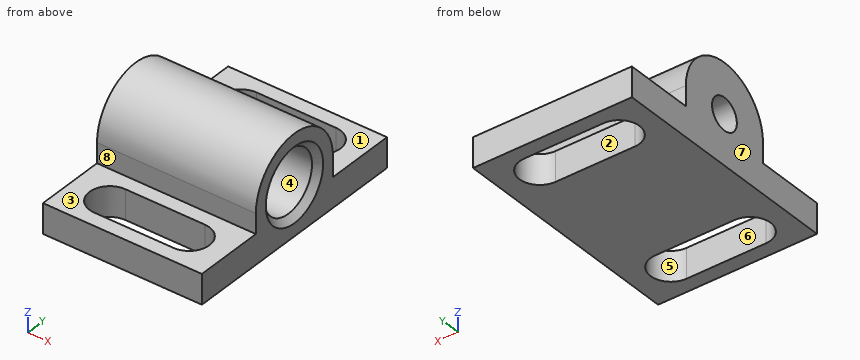
```python
from build123d import *

# Parameters (mm, degrees)
BOSS_EXTRUDE1_DEPTH = 25.4
CUT_EXTRUDE2_REACH  = 37.498


with BuildPart() as part:
    # Sketch1 → Boss-Extrude1 (new body)
    with BuildSketch(Plane(origin=(0, 0, 0), x_dir=(0, 0, -1), z_dir=(1, 0, 0))):
        with BuildLine():
            Line((0, -19.05), (0, 19.05))
            Line((0, 19.05), (-4.7498, 19.05))
            Line((-4.7498, 19.05), (-4.7498, 7.9375))
            Line((-4.7498, 7.9375), (-7.9375, 7.9375))
            ThreePointArc((-7.9375, 7.9375), (-15.875, 0), (-7.9375, -7.9375))
            Line((-7.9375, -7.9375), (-4.7498, -7.9375))
            Line((-4.7498, -7.9375), (-4.7498, -19.05))
            Line((-4.7498, -19.05), (0, -19.05))
        make_face()
    extrude(amount=-BOSS_EXTRUDE1_DEPTH)

    # Sketch2 → Cut-Revolve1 (revolve, cut)
    with BuildSketch(Plane(origin=(0, 0, 0), x_dir=(1, 0, 0), z_dir=(0, 1, 0)), mode=Mode.PRIVATE) as cut_revolve1_sk:
        Polygon((-25.4, -7.9375), (-25.4, -10.4902), (-19.05, -10.4902), (-19.05, -12.8397), (-1, -12.8397), (0, -13.8397), (0, -7.9375), align=None)
    revolve(cut_revolve1_sk.sketch.rotate(Axis((0, 0, 7.9375), (-1, 0, 0)), 180), axis=Axis((0, 0, 7.9375), (-1, 0, 0)), mode=Mode.SUBTRACT)

    # Sketch3 → Cut-Extrude2 (cut, up to next)
    with BuildSketch(Plane.XY, mode=Mode.PRIVATE) as cut_extrude2_sk1:
        with BuildLine():
            Line((-19.05, 16.7259), (-6.35, 16.7259))
            ThreePointArc((-6.35, 16.7259), (-3.1115, 13.4874), (-6.35, 10.2489))
            Line((-6.35, 10.2489), (-19.05, 10.2489))
            ThreePointArc((-19.05, 10.2489), (-22.2885, 13.4874), (-19.05, 16.7259))
        make_face()
    cut_extrude2_tool1 = extrude(cut_extrude2_sk1.sketch, amount=CUT_EXTRUDE2_REACH, mode=Mode.PRIVATE) & part.part
    # Sketch3 → Cut-Extrude2 (cut, up to next)
    with BuildSketch(Plane.XY, mode=Mode.PRIVATE) as cut_extrude2_sk2:
        with BuildLine():
            Line((-19.05, -16.7259), (-6.35, -16.7259))
            ThreePointArc((-6.35, -16.7259), (-3.1115, -13.4874), (-6.35, -10.2489))
            Line((-6.35, -10.2489), (-19.05, -10.2489))
            ThreePointArc((-19.05, -10.2489), (-22.2885, -13.4874), (-19.05, -16.7259))
        make_face()
    cut_extrude2_tool2 = extrude(cut_extrude2_sk2.sketch, amount=CUT_EXTRUDE2_REACH, mode=Mode.PRIVATE) & part.part
    add(cut_extrude2_tool1.solids().sort_by_distance((-12.7, 13.4874, 0))[0], mode=Mode.SUBTRACT)
    add(cut_extrude2_tool2.solids().sort_by_distance((-12.7, -13.4874, 0))[0], mode=Mode.SUBTRACT)


solid = part.part
```
The model under review builds one solid part; all positions refer to its coordinate system, in mm. Face numbers are marked on the shaded views. A direction names the side the tool comes from. Give positions to 0.01 mm unless a question says otherwise; leave off trailing zeros. Write each loop counter-clockwise with the first axis right and the second up, starting at its lowest first coordinate (ties: lowest second). Pieces come first, ordered by that corner, then holes. Notation, with made-up numbers: M -22,79.5 L 31,79.5 A22 ccw 31,97.5 Z; hole C 10,-8 d2. An arc over 180 degrees is marked long. Write item = value, one per line. Start each with the question number.
Q1. For line 1 (Y direction, x = -4, z = 3); line 2 (Y direction, x = -20, z = 10.25); line 3 (X direction, y = 2.5, z = 10.25), list the stretches that pass through material, from the lowest coordinate up.
Q2. Mouldability with a two-part tool opening along X and no side actions: class the marked faces 5, 6, 7 and 8 as released by +X, released by -X, zero draft, split by the parting line, or undercut.
Q3. We need section B-B (y = 0). State the section outline as (x, z) points (3 decimals), plus the area to 3 significant figures.
Q4. Clearance check with flat-ended pins moving along their axes: pin 1 (6 mm diameter, centred on x = -4, z = 5.5, fed in from +Y); pin 2 (3.5 mm diameter, centred on x = -18, z = 7, fed in from +Y); pin 3 (8 mm diameter, centred on x = -12.5, y = -7.5, fed in from +Z); pin 4 (3 mm diameter, centred on y = 0.5, z = 6.5, fed in from +X). State where each tip first meets the part, or that it passes through.
Q5. We need section A-A (x = -9.25). Give the number of separate pieces and of enclosed holes in the cut face, plus the area to 3 significant figures.
Q6. Machinability: for the marked faces 1, 2, 3 and 4, which of the approach directions +Z, -Z, +X, -X, +Y, -Y give a long, thin tool a straight path to every point of the face, cutting with its end or side? Answer none if there is none.
Q7. We need section D-D (z = 14.75). State the section outline as (x, y) points.
Result set:
q1.line_1 = -19.05 to -15.72, -11.26 to 11.26, 15.72 to 19.05
q1.line_2 = -7.59 to -1.08, 1.08 to 7.59
q1.line_3 = -25.4 to -19.05
q2.face_5 = undercut
q2.face_6 = undercut
q2.face_7 = released by -X
q2.face_8 = zero draft
q3.outline = M -25.4,0 L 0,0 L 0,2.035 L -1,3.035 L -19.05,3.035 L -19.05,5.385 L -25.4,5.385 Z; M -25.4,10.49 L -19.05,10.49 L -19.05,12.84 L -1,12.84 L 0,13.84 L 0,15.875 L -25.4,15.875 Z
q3.area = 183 mm2
q4.pin_1 = 19.05
q4.pin_2 = 7.94
q4.pin_3 = 15.06
q4.pin_4 = -19.05
q5.separate_pieces = 3
q5.enclosed_holes = 1
q5.area = 194 mm2
q6.face_1 = +Z, +X, -X, +Y
q6.face_2 = +Z, -Z
q6.face_3 = +Z, +X, -X, -Y
q6.face_4 = +X
q7.outline = M -25.4,-4.07 L 0,-4.07 L 0,4.07 L -25.4,4.07 Z
